The listing builds one solid part. Answer for the finished solid, in the listing's coordinates (mm). Face numbers are marked on the shaded views. A direction names the side the tool comes from. Give positions to 0.01 mm unless a question says otherwise; leave off trailing zeros. Order: outer loops, then holes, each group sorted by start corner. A loop starts at its lowest first (then second) coordinate and runs counter-clockwise, first axis right, second up. Notation, with made-up numbers: (-3.75, -15) - (46.25, -15) arc R32 ccw to (46.25, 14) - close; hole circle Ø2 at (75.5, -9). An arc over 180 degrees is marked (long way). Write each question's results on one line, items separated by ' | '. Start each with the question number.
1. Which of the six approach directions +Z, -Z, +X, -X, +Y, -Y give full straight-line access (tool end or side, diameter ignored) to the marked faces 5 and 6?
2. Find the intervals of material crossed by L1, parallel to Y at x = 0, z = 0.3; L2, parallel to X at y = 4.75, z = 0.55 (3 decimals); L3, parallel to X at y = 0, z = -0.3, in increasing order.
3. Section B-B (x = 0) is taken. Give the vertices of the cut face in (y, z) (1 decimal), and give its area (3 significant figures).
4. Determine the mould class of the marked faces 1, 2, 3 and 4 for opening direction X: released by +X, released by -X, zero draft, split by the parting line, or undercut.
5. Section A-A (y = 0) is taken. Give the vertices of the cut face in (x, z) (1 decimal), and give its area (3 significant figures).
6. Section D-D (y = 3.5) is taken. Give the vertices of the cut face in (x, z) (1 decimal), and give its area (3 significant figures).
7. Section C-C (z = 0.4) is taken. Give the vertices of the cut face in (x, y) (1 decimal).
Autodesk Inventor part; units mm, degrees
ref_plane "YZ Plane" through (0, 0, 0) normal (1, 0, 0) x (0, 1, 0)
ref_plane "XZ Plane" through (0, 0, 0) normal (0, 1, 0) x (-1, 0, 0)
ref_plane "XY Plane" through (0, 0, 0) normal (0, 0, 1) x (1, 0, 0)
sketch "Sketch1" plane through (0, 0, 0) normal (0, 0, 1) x (1, 0, 0)
  circle A0 centre (0, 0) radius 1.651 construction
  circle A1 centre (0, 4.7625) radius 1.0478
  arc A2 (1.905, 4.7625) -> (-1.905, 4.7625) centre (0, 4.7625) ccw
  line L0 (-1.905, 4.7625) -> (-1.905, 3.5178)
  line L1 (1.905, 4.7625) -> (1.905, 3.5178)
  arc A3 (-1.905, 3.5178) -> (-1.27, -3.7936) centre (0, 0) ccw
  line L2 (-1.27, -3.7936) -> (-1.27, -1.0549)
  line L3 (-6.0242, 0) -> (6.0242, 0) construction
  line L4 (0, -6.1357) -> (0, 8.8014) construction
  arc A4 (1.27, -3.7936) -> (1.905, 3.5178) centre (0, 0) ccw
  line L5 (1.27, -3.7936) -> (1.27, -1.0549)
  arc A5 (1.27, -1.0549) -> (-1.27, -1.0549) centre (0, 0) ccw
  dimension "d0" = 3.302
  dimension "d1" = 2.0955
  dimension "d2" = 4.7625
  dimension "d3" = 1.905
  dimension "d4" = 4.0005
  dimension "d5" = 2.54
extrude "Extrusion1" add sketch "Sketch1" along normal mid plane 1.27
fillet "Fillet1" radius 1.5875 2 edges at (1.905, 3.5178, 0) (-1.905, 3.5178, 0)
properties part number "Front Suspension Adjustment Clip"
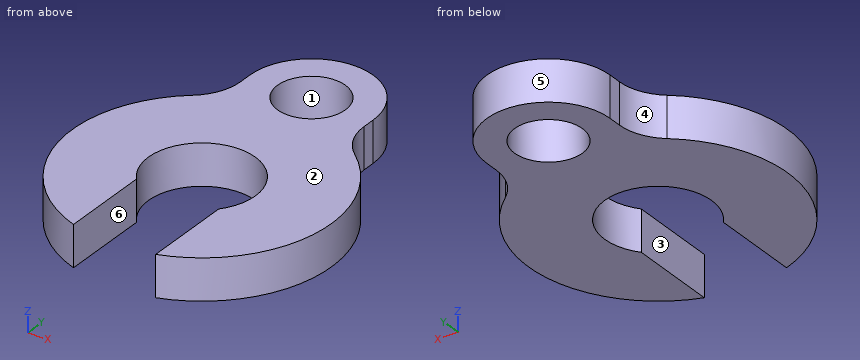
Reported:
1) face 5: +Z, -Z, +Y | face 6: +Z, -Z, -Y
2) L1: 1.65 to 3.71, 5.81 to 6.67 | L2: -1.905 to -1.048, 1.048 to 1.905 | L3: -4 to -1.65, 1.65 to 4
3) outline: (1.7, -0.6) - (3.7, -0.6) - (3.7, 0.6) - (1.7, 0.6) - close; (5.8, -0.6) - (6.7, -0.6) - (6.7, 0.6) - (5.8, 0.6) - close | area: 3.71 mm²
4) face 1: undercut | face 2: zero draft | face 3: undercut | face 4: released by -X
5) outline: (-4, -0.6) - (-1.7, -0.6) - (-1.7, 0.6) - (-4, 0.6) - close; (1.7, -0.6) - (4, -0.6) - (4, 0.6) - (1.7, 0.6) - close | area: 5.97 mm²
6) outline: (-2.2, -0.6) - (2.2, -0.6) - (2.2, 0.6) - (-2.2, 0.6) - close | area: 5.49 mm²
7) outline: (-2.5, 3.1) arc R4 ccw to (-1.3, -3.8) - (-1.3, -1.1) arc R1.7 cw (long way) to (1.3, -1.1) - (1.3, -3.8) arc R4 ccw to (2.5, 3.1) arc R1.6 cw to (1.9, 4.4) - (1.9, 4.8) arc R1.9 ccw to (-1.9, 4.8) - (-1.9, 4.4) arc R1.6 cw to start; hole circle Ø2.1 at (0, 4.8)
